```python
from build123d import *

# Parameters (mm, degrees)
F0_R     = 22.5
F0_R_2   = 9
F1_DEPTH = 45
F3_DEPTH = 6
F4_SIZE  = 0.5


# Not quite as in the source:
# - after a boolean that leaves OpenCascade's solid faulty, fix() repairs it


with BuildPart() as f1:
    # F0 (on Top) → F1 (new body)
    with BuildSketch(Plane.XY):
        Circle(F0_R)
        Circle(F0_R_2, mode=Mode.SUBTRACT)
    extrude(amount=F1_DEPTH)

    # F2 (on face) → F3 (join)
    with BuildSketch(Plane.XY.offset(45)):
        with BuildLine():
            ThreePointArc((-21.6852484422, 6), (-22.5, 0), (-21.6852484422, -6))
            Line((-21.6852484422, -6), (-9.2195444573, -6))
            Line((-9.2195444573, -6), (-7.5432636469, -4.9090909091))
            ThreePointArc((-7.5432636469, -4.9090909091), (-9, 0), (-7.5432636469, 4.9090909091))
            Line((-7.5432636469, 4.9090909091), (-9.2195444573, 6))
            Line((-9.2195444573, 6), (-21.6852484422, 6))
        make_face()
        with BuildLine():
            ThreePointArc((6, 21.6852484422), (0, 22.5), (-6, 21.6852484422))
            Line((-6, 21.6852484422), (-6, 9.2195444573))
            Line((-6, 9.2195444573), (-4.9090909091, 7.5432636469))
            ThreePointArc((-4.9090909091, 7.5432636469), (0, 9), (4.9090909091, 7.5432636469))
            Line((4.9090909091, 7.5432636469), (6, 9.2195444573))
            Line((6, 9.2195444573), (6, 21.6852484422))
        make_face()
        with BuildLine():
            Line((9.2195444573, -6), (21.6852484422, -6))
            ThreePointArc((21.6852484422, -6), (22.2953816961, -3.0275328281), (22.5, 0))
            ThreePointArc((22.5, 0), (22.2953816961, 3.0275328281), (21.6852484422, 6))
            Line((21.6852484422, 6), (9.2195444573, 6))
            Line((9.2195444573, 6), (7.5432636469, 4.9090909091))
            ThreePointArc((7.5432636469, 4.9090909091), (8.6281334257, 2.5603346635), (9, 0))
            ThreePointArc((9, 0), (8.6281334257, -2.5603346635), (7.5432636469, -4.9090909091))
            Line((7.5432636469, -4.9090909091), (9.2195444573, -6))
        make_face()
        with BuildLine():
            Line((-6, -9.2195444573), (-6, -21.6852484422))
            ThreePointArc((-6, -21.6852484422), (0, -22.5), (6, -21.6852484422))
            Line((6, -21.6852484422), (6, -9.2195444573))
            Line((6, -9.2195444573), (4.9090909091, -7.5432636469))
            ThreePointArc((4.9090909091, -7.5432636469), (0, -9), (-4.9090909091, -7.5432636469))
            Line((-4.9090909091, -7.5432636469), (-6, -9.2195444573))
        make_face()
    extrude(amount=F3_DEPTH)

    add(f1.part.fix(), mode=Mode.REPLACE)

    # F4
    f4_edges = [f1.edges().sort_by_distance(p)[0] for p in [
        (-22.5, 0, 51),
        (0, 22.5, 51),
        (22.5, 0, 51),
        (0, -22.5, 51),
    ]]
    chamfer(f4_edges, length=F4_SIZE)


solid = f1.part
```
Work out the finished part from the listing and answer in its coordinate system (mm). A direction names the side the tool comes from. Round coordinates to 2 decimals unless told otherwise and drop trailing zeros. Write each loop counter-clockwise with the first axis right and the second up, starting at its lowest first coordinate (ties: lowest second). Pieces come first, ordered by that corner, then holes. Notation, with made-up numbers: (46.5, -33.75) - (104.5, -33.75) arc R33 cw to (104.5, 1.25) - close; hole circle Ø4 at (10.5, 0). An arc over 180 degrees is marked (long way). Return JSON: item names as keys, results as strings. Group by question number.
Q1. The part is cut by section D-D on x = 20. Write down the section's boundary in (y, z), then the cut area to 4 significant figures.
Q2. The part is cut by section C-C on z = 27.5. Write down the section's boundary in (x, y).
Q3. The mould has two halves that part along X. Classify faces 6 (the flat face through (-8.39, -5.46, 47.96)), 7 (the flat face through (8.39, 5.46, 47.96)), 8 (the flat face through (5.447, 8.37, 47.958)), 9 (the flat face through (-5.46, 8.39, 47.96)): released by +X, released by -X, zero draft, split by the parting line, or undercut.
Q4. The part is cut by section A-A on x = 0. Write down the section's boundary in (y, z).
Q5. For faces 1 (the flat face through (-8.37, 5.447, 47.958)), 2 (the flat face through (-6, 16, 48)), 3 (the flat face through (6, 15, 48)), 4 (the flat face through (5.46, -8.39, 47.96)), 5 (the flat face through (-15, 6, 48)), determine the directions among +Z, -Z, +X, -X, +Y, -Y from which every point of the face is accessible in a straight line to the end or side of a thin tool.
Q6. The part is cut by section B-B on y = -13.5. Write down the section's boundary in (x, z), then the cut area to 3 significant figures.
Q7. Each of these flat-tipped pins is pushed along its axis until it touches: pin 1 Ø1.8 at (y, z) = (-15, 48.5) entering from -X; pin 2 Ø5 at (x, z) = (-11, 14) entering from -Y; pin 3 Ø3 at (y, z) = (-15, 48.5) entering from +X. Where does it stop, or does it pass through?
Q8. Find the intervals of material crossed by L1, parallel to X at y = 0, z = 20.5; L2, parallel to Z at x = 16, y = -8.5, in increasing order.
Solved:
{
 "1": {"outline": "(-10.31, 0) - (10.31, 0) - (10.31, 45) - (6, 45) - (6, 51) - (-6, 51) - (-6, 45) - (-10.31, 45) - close", "area": "1,000 mm²"},
 "2": {"outline": "circle Ø45 at (0, 0); hole circle Ø18 at (0, 0)"},
 "3": {"face 6": "undercut", "face 7": "undercut", "face 8": "released by +X", "face 9": "released by -X"},
 "4": {"outline": "(-22.5, 0) - (-9, 0) - (-9, 51) - (-22, 51) - (-22.5, 50.5) - close; (9, 0) - (22.5, 0) - (22.5, 50.5) - (22, 51) - (9, 51) - close"},
 "5": {"face 1": "+Z, +Y", "face 2": "+Z, -X, +Y, -Y", "face 3": "+Z, +X, +Y, -Y", "face 4": "+Z, +X", "face 5": "+Z, +X, -X, +Y"},
 "6": {"outline": "(-18, 0) - (18, 0) - (18, 45) - (6, 45) - (6, 51) - (-6, 51) - (-6, 45) - (-18, 45) - close", "area": "1,690 mm²"},
 "7": {"pin 1": "x = -6", "pin 2": "y = -20.83", "pin 3": "x = 6"},
 "8": {"L1": "-22.5 to -9, 9 to 22.5", "L2": "0 to 45"}
}
